CAD build for the part. Positions are in the model's coordinates, mm. A direction names the side the tool comes from. Give positions to 0.01 mm unless a question says otherwise; leave off trailing zeros. Loops run counter-clockwise (first coordinate to the right, second up) from the corner with the lowest first, then second, coordinate; pieces in that order, holes last. Notation, with made-up numbers: M 75,25 L 133,25 A17 cw 133,44 Z; hole C 49,-27.75 d11. An arc over 180 degrees is marked long. Answer as CSV lines item,"result".
from build123d import *

# Parameters (mm, degrees)
F0_R     = 65.4726096666
F1_DEPTH = 38.1
F2_R     = 52.6067732991
F3_DEPTH = 25.4
F4_R     = 35.1837218131
F5_DEPTH = 25.4


# Not quite as in the source:
# - the program builds the solid bodies; features that only make, move or delete a surface that nothing else refers to are left out


with BuildPart() as f1:
    # F0 (on Top) → F1 (new body)
    with BuildSketch(Plane.XY):
        Circle(F0_R)
    extrude(amount=F1_DEPTH)

    # F2 (on face) → F3 (join)
    with BuildSketch(Plane.XY.offset(38.1)):
        Circle(F2_R)
    extrude(amount=F3_DEPTH)

    # F4 (on face) → F5 (join)
    with BuildSketch(Plane.XY.offset(63.5)):
        Circle(F4_R)
    extrude(amount=F5_DEPTH)


solid = f1.part
1) Flat gauge pins, fed straight in: pin 1 (6 mm diameter, centred on y = -36.5, z = 40, fed in from +X); pin 2 (12 mm diameter, centred on y = -11, z = 64, fed in from -X); pin 3 (4 mm diameter, centred on x = -10, z = 16.5, fed in from +Y). Where does each tip first touch, or does it go through?
Answer below:
pin 1,"stops at x = 55.84"
pin 2,"stops at x = -52.37"
pin 3,"stops at y = 64.98"
2) Band-saw the part on A-A on y = 0. Give the cut face in (x, z), and give its area (3 significant figures).
Answer below:
outline,"M -65.47,0 L 65.47,0 L 65.47,38.1 L 52.61,38.1 L 52.61,63.5 L 35.18,63.5 L 35.18,88.9 L -35.18,88.9 L -35.18,63.5 L -52.61,63.5 L -52.61,38.1 L -65.47,38.1 Z"
area,"9,450 mm^2"
3) Band-saw the part on D-D on x = 43. Give the cut face in (y, z).
Answer below:
outline,"M -49.37,0 L 49.37,0 L 49.37,38.1 L 30.31,38.1 L 30.31,63.5 L -30.31,63.5 L -30.31,38.1 L -49.37,38.1 Z"
4) Mould opens along X. For faces 3 (the face through (34, -11, 63.5)), 4 (the face through (62.45, 19.67, 18.78)) say: +X half, -X half, draft (parallel to the pull), parting line (faces both ways), or undercut.
Answer below:
face 3,"draft"
face 4,"parting line"
5) Drill centre lines: line 1 (Z direction, x = -5, y = -37.5); line 2 (Z direction, x = -35.5, y = 49); line 3 (Y direction, x = 22, z = 50). Where is each one in solid material? Low to high. Write a range as from..to.
Answer below:
line 1,"z = 0..63.5"
line 2,"z = 0..38.1"
line 3,"y = -47.79..47.79"
6) Band-saw the part on C-C on z = 35. Give the cut face in (x, y), and give its area (3 significant figures).
Answer below:
outline,"C 0,0 d130.95"
area,"13,500 mm^2"
7) Which spindle directions (+Z, -Z, +X, -X, +Y, -Y) get a long thin tool onto all of the face, cutting with end or side? Do faces 1 (the face through (24.275, -46.671, 50.622)), 2 (the face through (0, 0, 88.9)). Say none if no direction does.
Answer below:
face 1,"+Z"
face 2,"+Z, +X, -X, +Y, -Y"
